from build123d import *

# Parameters (mm, degrees)
EXTRUDE_1_DEPTH = 5
SKETCH_3_W      = 8.851756477
SKETCH_3_H      = 8.100037161
EXTRUDE_2_DEPTH = 95
SKETCH_7_R      = 0.8
EXTRUDE_3_DEPTH = 5


with BuildPart() as part:
    # 草图1 → 凸台-拉伸1 (new body)
    with BuildSketch(Plane.XY):
        with BuildLine():
            ThreePointArc((-9.310291372, -5.5207396), (-9.401635933, -5.061519481), (-9.661763234, -4.672211463))
            Line((-9.661763234, -4.672211463), (-10.510291372, -5.5207396))
            Line((-10.510291372, -5.5207396), (-9.661763234, -6.369267738))
            ThreePointArc((-9.661763234, -6.369267738), (-9.401635933, -5.979959719), (-9.310291372, -5.5207396))
        make_face()
        with BuildLine():
            Line((-10.510291372, -5.5207396), (-9.661763234, -4.672211463))
            ThreePointArc((-9.661763234, -4.672211463), (-10.510291372, -4.3207396), (-11.358819509, -4.672211463))
            Line((-11.358819509, -4.672211463), (-10.510291372, -5.5207396))
        make_face()
        with BuildLine():
            Line((-9.661763234, -6.369267738), (-10.510291372, -5.5207396))
            Line((-10.510291372, -5.5207396), (-11.358819509, -6.369267738))
            ThreePointArc((-11.358819509, -6.369267738), (-10.510291372, -6.7207396), (-9.661763234, -6.369267738))
        make_face()
        with BuildLine():
            Line((-11.358819509, -6.369267738), (-10.510291372, -5.5207396))
            Line((-10.510291372, -5.5207396), (-11.358819509, -4.672211463))
            ThreePointArc((-11.358819509, -4.672211463), (-11.710291372, -5.5207396), (-11.358819509, -6.369267738))
        make_face()
    extrude(amount=EXTRUDE_1_DEPTH)

    # 草图2 → 旋转2 (revolve)
    with BuildSketch(Plane.XY.offset(5)):
        with BuildLine():
            Line((-7.264243744, -2.550356662), (-13.756338999, -8.491122538))
            ThreePointArc((-13.756338999, -8.491122538), (-7.539908434, -8.766787228), (-7.264243744, -2.550356662))
        make_face()
    revolve(axis=Axis((-7.264243744, -2.550356662, 5), (-0.737738097, -0.675087031, 0)))

    # 草图3 → 凸台-拉伸2 (add)
    with BuildSketch(Plane(origin=(0, 0, 0), x_dir=(-1, 0, 0), z_dir=(0, 0, -1))):
        with Locations((10.510291371, -5.520739601)):
            Rectangle(SKETCH_3_W, SKETCH_3_H)
    extrude(amount=EXTRUDE_2_DEPTH)

    # 草图7 → 凸台-拉伸3 (add)
    with BuildSketch(Plane(origin=(0, 0, -95), x_dir=(-1, 0, 0), z_dir=(0, 0, -1))):
        with Locations((10.510291372, -5.5207396)):
            Circle(SKETCH_7_R)
    extrude(amount=EXTRUDE_3_DEPTH)

    # 草图5 one side → 旋转4 (revolve)
    with BuildSketch(Plane(origin=(0, 0, -100), x_dir=(-1, 0, 0), z_dir=(0, 0, -1))):
        with BuildLine():
            ThreePointArc((9.920100894, -6.060809225), (10.799987435, -6.266444764), (11.310291372, -5.5207396))
            ThreePointArc((11.310291372, -5.5207396), (11.255996535, -5.231043537), (11.100481849, -4.980669975))
            Line((11.100481849, -4.980669975), (9.920100894, -6.060809225))
        make_face()
        with BuildLine():
            ThreePointArc((7.264243744, -8.491122538), (13.48067431, -8.766787228), (13.756338999, -2.550356662))
            Line((13.756338999, -2.550356662), (7.264243744, -8.491122538))
        make_face()
    revolve(axis=Axis((-13.756338999, -2.550356662, -100), (0.737738097, -0.675087031, 0)))


solid = part.part
For this review, take the finished solid that the model builds, in its own axes (mm). A direction names the side the tool comes from. Round coordinates to 2 decimals unless told otherwise and drop trailing zeros. Loops run counter-clockwise (first coordinate to the right, second up) from the corner with the lowest first, then second, coordinate; pieces in that order, holes last. Notation, with made-up numbers: (-28, 55) - (-20, 55) arc R5 cw to (-20, 61) - close; hole circle Ø4 at (17.5, 32.25). An arc over 180 degrees is marked (long way). One line per item, written item: value. Start each with the question number.
Item 1: Clearance check with flat-ended pins moving along their axes: pin 1 Ø5 at (x, y) = (-14, -4.5) entering from +Z; pin 2 Ø4 at (x, y) = (-9.5, -8) entering from -Z; pin 3 Ø2.5 at (x, z) = (-12, -59.5) entering from +Y. State where each tip first meets the part, or that it passes through.
Item 2: For L1, parallel to Z at x = -12, y = -2.5; L2, parallel to Z at x = -14.25, y = -6.5; L3, parallel to Z at x = -14, y = -8.75, list the stretches that pass through material, from the lowest coordinate up.
Item 3: Take a section at B-B (z = -3). Give the boundary of the cut face in (x, y).
Item 4: The part is to be moulded in two halves that separate along Z. For faces 3 (the flat face through (-14.936, -6, -47)), 4 (the flat face through (-9, -6, 0)), 5 (the flat face through (-10, -9.571, -47)), say which applies: +Z half, -Z half, draft (parallel to the pull), parting line (faces both ways), or undercut.
Item 5: For faces 1 (the flat face through (-6.084, -6, -47)), 2 (the flat face through (-10, -1.471, -47)), list the 3-axis set-ups (+Z, -Z, +X, -X, +Y, -Y) from which the entire face can be reached by the end or side of a thin tool; tool diameter is ignored.
Item 6: Take a section at A-A (x = -8.25). Give the boundary of the cut face in (y, z).
Answer below:
1. pin 1: stops at z = 9.25
1. pin 2: stops at z = -104.35
1. pin 3: stops at y = -1.47
2. L1: z = -102.83 to -97.17, -95 to 0, 2.17 to 7.83
2. L2: z = -102.1 to -97.9, -95 to 0, 2.9 to 7.1
2. L3: z = -95 to 0
3. outline: (-14.94, -9.57) - (-6.08, -9.57) - (-6.08, -1.47) - (-14.94, -1.47) - close
4. face 3: draft
4. face 4: undercut
4. face 5: undercut
5. face 1: +Z, -Z, +X, +Y, -Y
5. face 2: +X, -X, +Y
6. outline: (-9.57, -95) - (-1.47, -95) - (-1.47, 0) - (-9.57, 0) - close; circle Ø7.55 at (-5.52, -100); circle Ø7.55 at (-5.52, 5)
